Geometry check sheet. Reference: the model listing, model coordinates, mm. A direction names the side the tool comes from. Round coordinates to 2 decimals unless told otherwise and drop trailing zeros. Order: outer loops, then holes, each group sorted by start corner. A loop starts at its lowest first (then second) coordinate and runs counter-clockwise, first axis right, second up. Notation, with made-up numbers: (38, -32) -> (62, -32) arc R21 cw to (62, -2) -> close; hole circle Ø6 at (51.25, -32.75). An arc over 180 degrees is marked (long way). Use a Markdown table: item, result. Add a question column.
Item 1: Material ranges on probe 1 along Z at (x, y) = (1, 5); probe 2 along X at (y, z) = (1.75, -4.5); probe 3 along Y at (x, z) = (8.5, 0.25), recorded low to high. Write a range as [from, to].
Item 2: Mould release check, pull along Y, two halves, no side actions. Record for faces 4 (the flat face through (0.852, -3.814, -4.868)), 5 (the flat face through (1.727, -4.5, -2)), 6 (the conical face through (0.85, 4.98, -5)): pulls with the +Y half, pulls with the -Y half, needs draft (parallel to the pull), parting line crosses it, or undercut.
Item 3: Set-up check for faces 1 (the cylindrical face through (0.85, 5.01, 2.05)), 2 (the cylindrical face through (0.85, 2.05, -5.01)), 3 (the cylindrical face through (0.85, -2.05, 5.01)): record each of +Z, -Z, +X, -X, +Y, -Y from which the full face is reachable in a straight line by a thin tool's end or side.
Item 4: Gauge pin test, flat ends, axial feed: pin 1 Ø2 at (x, z) = (13.5, -3) entering from +Y; pin 2 Ø1.5 at (x, z) = (7.5, -5) entering from -Y; pin 3 Ø1.4 at (x, y) = (1, 6) entering from +Z. Record the tip position at first contact, or that the pin passes through.
Item 5: Sectioned sample at D-D, the plane x = -0.5. Record the cut outline in (y, z), and give its area (3 significant figures).
Item 6: Sectioned sample at C-C, the plane x = 20. Record the cut outline in (y, z) (1 decimal), and give its area (3 significant figures).
from build123d import *

# Parameters (mm, degrees)
RIBCUT_START     = -1.7272
RIBCUT_DEPTH     = 1.7272
RIBCUTSPAT_COUNT = 8
RIBCUTSPAT_ANGLE = 315


with BuildPart() as part:
    # BodySke → BaseBody (revolve)
    with BuildSketch(Plane.XY, mode=Mode.PRIVATE) as basebody_sk:
        with BuildLine():
            Line((-2.159, 6.9342), (-2.159, 0))
            Line((-2.159, 0), (25.4, 0))
            Line((25.4, 0), (25.4, 3.81635))
            Line((25.4, 3.81635), (24.45385, 4.7625))
            Line((24.45385, 4.7625), (1.7272, 4.7625))
            Line((1.7272, 4.7625), (1.7272, 6.735735096))
            Line((1.7272, 6.735735096), (0.00254, 7.36346))
            Line((0.00254, 7.36346), (0, 7.36346))
            Line((0, 7.36346), (0, 7.366))
            Line((0, 7.366), (-1.7272, 7.366))
            ThreePointArc((-1.7272, 7.366), (-2.032528708, 7.239528708), (-2.159, 6.9342))
        make_face()
    revolve(basebody_sk.sketch.rotate(Axis((0, 0, 0), (1, 0, 0)), 90), axis=Axis((0, 0, 0), (1, 0, 0)))

    # RibCutSke → RibCut (cut)
    with BuildSketch(Plane(origin=(1.7272, 1.794401132, -0.090952894), x_dir=(0, 0, -1), z_dir=(1, 0, 0)).offset(RIBCUT_START)):
        with BuildLine():
            Line((0.654066246, 3.567461918), (0.654066246, 5.533825289))
            ThreePointArc((0.654066246, 5.533825289), (2.727893269, 5.010895504), (4.564077617, 3.91424555))
            Line((4.564077617, 3.91424555), (3.173648743, 2.523816676))
            ThreePointArc((3.173648743, 2.523816676), (1.980656032, 3.206905232), (0.654066246, 3.567461918))
        make_face()
    ribcut = extrude(amount=RIBCUT_DEPTH, mode=Mode.SUBTRACT)

    # RibCutsPat: RibCut ×8 about axis
    ribcutspat_axis = Axis((0, 0, 0), (1, 0, 0))
    for i in range(1, RIBCUTSPAT_COUNT):
        add(ribcut.rotate(ribcutspat_axis, i * RIBCUTSPAT_ANGLE / (RIBCUTSPAT_COUNT - 1)), mode=Mode.SUBTRACT)


solid = part.part
Found:
| question | item | result |
|---|---|---|
| 1 | probe 1 | z = [-4.9, -3.95], [-2.07, 2.07], [3.95, 4.9] |
| 1 | probe 2 | x = [-2.16, 1.73] |
| 1 | probe 3 | y = [-4.76, 4.76] |
| 2 | face 4 | undercut |
| 2 | face 5 | needs draft |
| 2 | face 6 | pulls with the +Y half |
| 3 | face 1 | +X, +Y |
| 3 | face 2 | -Z, +X |
| 3 | face 3 | +Z, +X |
| 4 | pin 1 | stops at y = 4.32 |
| 4 | pin 2 | stops at y = -2.15 |
| 4 | pin 3 | stops at z = 4.66 |
| 5 | outline | circle Ø14.73 at (0, 0) |
| 5 | area | 170 mm2 |
| 6 | outline | circle Ø9.5 at (0, 0) |
| 6 | area | 71.3 mm2 |
